Design review of the part built by this model. Coordinates are the model's own, in mm. A direction names the side the tool comes from. Round coordinates to 2 decimals unless told otherwise and drop trailing zeros. Order: outer loops, then holes, each group sorted by start corner. A loop starts at its lowest first (then second) coordinate and runs counter-clockwise, first axis right, second up. Notation, with made-up numbers: (-13.75, -33.5) - (35.25, -33.5) arc R23 cw to (35.25, -11.5) - close; hole circle Ø8 at (-31, -30). An arc over 180 degrees is marked (long way). Use CSV: the item, a comma, the result in double quotes. Start each with the question number.
Autodesk Inventor part; units mm, degrees
ref_plane "YZ Plane" through (0, 0, 0) normal (1, 0, 0) x (0, 1, 0)
ref_plane "XZ Plane" through (0, 0, 0) normal (0, 1, 0) x (-1, 0, 0)
ref_plane "XY Plane" through (0, 0, 0) normal (0, 0, 1) x (1, 0, 0)
sketch "Sketch1" plane through (0, 0, 0) normal (0, 0, 1) x (1, 0, 0)
  circle A0 centre (0, 0) radius 1
  dimension "d0" = 2
extrude "Extrusion1" add sketch "Sketch1" along normal blind 8
sketch "Sketch2" plane through (0, 0, 0) normal (0, 0, -1) x (-1, 0, 0)
  circle A0 centre (0, 0) radius 1.75
  dimension "d3" = 3.5
extrude "Extrusion2" add sketch "Sketch2" along normal blind 1
sketch "Sketch3" plane through (0, 0, -1) normal (0, 0, -1) x (-1, 0, 0)
  circle A0 centre (0, 0) radius 1
  line L0 (-0.2879, -0.9577) -> (0.2879, -0.9577)
  line L1 (0.2879, -0.9577) -> (0.2879, 0.9577)
  line L2 (0.2879, 0.9577) -> (-0.2879, 0.9577)
  line L3 (-0.2879, 0.9577) -> (-0.2879, -0.9577)
  line L4 (-0.2879, -0.9577) -> (0.2879, 0.9577) construction
  line L5 (0.2879, -0.9577) -> (-0.2879, 0.9577) construction
  line L6 (-0.9577, 0.2879) -> (0.9577, 0.2879)
  line L7 (0.9577, 0.2879) -> (0.9577, -0.2879)
  line L8 (0.9577, -0.2879) -> (-0.9577, -0.2879)
  line L9 (-0.9577, -0.2879) -> (-0.9577, 0.2879)
  line L10 (-0.9577, 0.2879) -> (0.9577, -0.2879) construction
  line L11 (0.9577, 0.2879) -> (-0.9577, -0.2879) construction
extrude "Extrusion3" cut sketch "Sketch3" against normal blind 0.5 contours L7 L8 L1 L6 | L1 L6 L3 L2 | L1 L8 L3 L6 | L0 L3 L8 L1 | L3 L8 L9 L6
fillet "Fillet1" radius 0.6 1 edges at (1.75, 0, -1)
fillet "Fillet2" radius 0.1 1 edges at (-1, 0, 8)
properties part number "M2"
Q1. Clearance check with a flat-ended pin moving along its axis: pin 1 (0.6 mm diameter, centred on y = 0.5, z = -0.5, fed in from +X). State where the tip first meets the part, or that it passes through.
Q2. For L1, parallel to Z at x = -0.8, y = -0.65; L2, parallel to Z at x = 0.2, y = 0.1; L3, parallel to X at y = -0.05, z = 4.75, list the stretches that pass through material, from the lowest coordinate up. Write a range as [from, to].
Q3. Take a section at A-A (x = 0). State the section outline as (y, z) points, plus the area to 3 significant figures.
Q4. Tool access review of faces 4 (the flat face through (0, 0, 8)), 5 (the flat face through (-1, -1, 0)): name each direction out of +Z, -Z, +X, -X, +Y, -Y from which nothing blocks a thin tool from reaching the whole face with its end or side.
Q5. Take a section at C-C (z = 2.25). State the section outline as (x, y) points, plus the area to 3 significant figures.
Q6. The part is to be moulded in two halves that separate along X. For faces 1 (the cylindrical face through (-1.617, 0.67, -0.197)), 2 (the flat face through (0, 0, -0.5)), 3 (the flat face through (-0.5, -0.5, -1)), say which applies: +X half, -X half, draft (parallel to the pull), parting line (faces both ways), or undercut.
Findings below:
1,pin 1,"stops at x = 1.74"
2,L1,"z = [-1, 0]"
2,L2,"z = [-0.5, 8]"
2,L3,"x = [-1, 1]"
3,outline,"(-1.75, -0.4) arc R0.6 ccw to (-1.15, -1) - (-0.96, -1) - (-0.96, -0.5) - (0.96, -0.5) - (0.96, -1) - (1.15, -1) arc R0.6 ccw to (1.75, -0.4) - (1.75, 0) - (1, 0) - (1, 7.9) arc R0.1 ccw to (0.9, 8) - (-0.9, 8) arc R0.1 ccw to (-1, 7.9) - (-1, 0) - (-1.75, 0) - close"
3,area,"18.4 mm^2"
4,face 4,"+Z, +X, -X, +Y, -Y"
4,face 5,"+Z"
5,outline,"circle Ø2 at (0, 0)"
5,area,"3.14 mm^2"
6,face 1,"parting line"
6,face 2,"undercut"
6,face 3,"draft"
